from build123d import *

# Parameters (mm, degrees)
EXTRUDE_1_DEPTH        = 90
HOLE_WIZARD_M6_1_D     = 5
HOLE_WIZARD_M6_1_DEPTH = 28
HOLE_WIZARD_M6_1_TIP   = 1.502151548


with BuildPart() as part:
    # 草图1 → 凸台-拉伸1 (new, symmetric)
    with BuildSketch(Plane(origin=(0, 0, 0), x_dir=(0, 0, -1), z_dir=(1, 0, 0))):
        Polygon((-4.1, 13.85), (-4.1, 2.05), (-2.05, 0), (0, 0), (0, 4), (1.8, 4), (1.8, 11.9), (0, 11.9), (0, 15.9), (-2.05, 15.9), align=None)
    extrude(amount=EXTRUDE_1_DEPTH, both=True)

    # M6 螺纹孔1
    with Locations(Plane(origin=(70, 7.95, -1.8), x_dir=(-1, 0, 0), z_dir=(0, 0, -1))):
        with Locations((0, 0), (49.75, 0), (90.25, 0), (140, 0)):
            Hole(HOLE_WIZARD_M6_1_D / 2, depth=HOLE_WIZARD_M6_1_DEPTH)
            with Locations((0, 0, -(HOLE_WIZARD_M6_1_DEPTH + HOLE_WIZARD_M6_1_TIP / 2))):  # 118° drill point
                Cone(0, HOLE_WIZARD_M6_1_D / 2, HOLE_WIZARD_M6_1_TIP, mode=Mode.SUBTRACT)


solid = part.part
Here's how the part is built. I have some questions about the finished solid (model axes, mm). A direction names the side the tool comes from. Coordinates: 2 decimals unless noted, no trailing zeros. Order: outer loops, then holes, each group sorted by start corner. A loop starts at its lowest first (then second) coordinate and runs counter-clockwise, first axis right, second up. Notation, with made-up numbers: M -11.5,0.25 L -1.5,0.25 A28 cw -1.5,38.25 Z; hole C -12.5,86 d10. An arc over 180 degrees is marked long. Answer as CSV lines item,"result". Start each with the question number.
1. I need wall thicknesses on line 1 (Y direction, x = -70, z = 0.2); line 2 (X direction, y = 9.75, z = 0.4); line 3 (Y direction, x = -59, z = -0.9). Which ranges of each line are inside material? Lowest first, please. Write a range as [from, to].
2. I want a section at B-B, the plane x = -20.25. Write out the boundary of the cut face in (y, z), and give its area (3 significant figures).
3. For pin 1 (2 mm diameter, centred on x = -38.5, y = 2.5, fed in from -Z); pin 2 (0.5 mm diameter, centred on x = 26, z = -0.5, fed in from +Y); pin 3 (0.5 mm diameter, centred on x = 4, z = -1.5, fed in from -Y), each with a flat end and sliding along its axis, tell me the tip position at first contact or that it passes through.
4. On a 3-axis mill with a long thin cutter (end or side, diameter ignored), from which of +Z, -Z, +X, -X, +Y, -Y can I reach the whole of each face in a straight line? I mean faces 1 (the cylindrical face through (-71.984, 6.429, 1.191)), 2 (the flat face through (1, 14, 0)). Say none if no direction works.
5. I want a section at C-C, the plane x = -59.5. Write out the boundary of the cut face in (y, z).
6. I want a section at A-A, the plane y = 7.95. Write out the boundary of the cut face in (x, z), and give its area (3 significant figures).
7. We'd pull the mould along X, two halves only. Please class faces 3 (the cylindrical face through (-22.748, 8.06, 1.191)), 4 (the flat face through (-90, 8, 1)), 5 (the flat face through (1, 2, 0)): released by +X, released by -X, zero draft, split by the parting line, or undercut.
Recorded:
1,line 1,"y = [0, 5.45], [10.45, 15.9]"
1,line 2,"x = [-90, -71.73], [-68.27, -21.98], [-18.52, 18.52], [21.98, 68.27], [71.73, 90]"
1,line 3,"y = [4, 11.9]"
2,outline,"M 0,0 L 4,0 L 4,-1.8 L 5.45,-1.8 L 5.45,4.1 L 2.05,4.1 L 0,2.05 Z; M 10.45,-1.8 L 11.9,-1.8 L 11.9,0 L 15.9,0 L 15.9,2.05 L 13.85,4.1 L 10.45,4.1 Z"
2,area,"45.7 mm2"
3,pin 1,"stops at z = 0"
3,pin 2,"stops at y = 11.9"
3,pin 3,"stops at y = 4"
4,face 1,"+Z, -Z"
4,face 2,"-Z, +X, -X, +Y"
5,outline,"M 0,0 L 4,0 L 4,-1.8 L 11.9,-1.8 L 11.9,0 L 15.9,0 L 15.9,2.05 L 13.85,4.1 L 2.05,4.1 L 0,2.05 Z"
6,outline,"M -90,-1.8 L -72.5,-1.8 L -72.5,4.1 L -90,4.1 Z; M -67.5,-1.8 L -22.75,-1.8 L -22.75,4.1 L -67.5,4.1 Z; M -17.75,-1.8 L 17.75,-1.8 L 17.75,4.1 L -17.75,4.1 Z; M 22.75,-1.8 L 67.5,-1.8 L 67.5,4.1 L 22.75,4.1 Z; M 72.5,-1.8 L 90,-1.8 L 90,4.1 L 72.5,4.1 Z"
6,area,"944 mm2"
7,face 3,"undercut"
7,face 4,"released by -X"
7,face 5,"zero draft"
